For this review, take the finished solid that the model builds, in its own axes (mm). Face numbers are marked on the shaded views. A direction names the side the tool comes from. Round coordinates to 2 decimals unless told otherwise and drop trailing zeros. Loops run counter-clockwise (first coordinate to the right, second up) from the corner with the lowest first, then second, coordinate; pieces in that order, holes last.
1) Take a section at A-A (x = 77). State the section outline as (y, z) points (3 decimals).
2) Wall thickness on L1, parallel to X at y = 203, z = 24.5; L2, parallel to Z at x = 143, y = 218.5; L3, parallel to Y at x = 37, z = 125.5: over which ranges is each line inside the solid? List them lowest first.
3) Insertion check: pin 1 (2 mm diameter, centred on x = 94.5, z = 6.5, fed in from -Y); pin 2 (12 mm diameter, centred on x = 132, y = 16.5, fed in from -Z); pin 3 (4 mm diameter, centred on x = 144, y = 40.5, fed in from -Z). Each pin has a flat end and moves straight along its axis. Give the tip position at first contact, or say it passes through.
4) Mouldability with a two-part tool opening along X and no side actions: class the marked faces 1, 2 and 3 as pulls with the +X half, pulls with the -X half, needs draft (parallel to the pull), parting line crosses it, or undercut.
5) Take a section at C-C (z = 112.5). State the section outline as (x, y) points, then the cut area to 3 significant figures.
6) Take a section at B-B (z = 40). State the section outline as (x, y) points.
7) Take a section at D-D (y = 0). State the section outline as (x, z) points.
8) Tool access review of the marked faces 4, 5 and 6: name each direction out of +Z, -Z, +X, -X, +Y, -Y from which nothing blocks a thin tool from reaching the whole face with its end or side.
```python
from build123d import *

# Parameters (mm, degrees)
F0_R      = 9.5
F1_DEPTH  = 291
F3_DEPTH  = 60
F4_DEPTH  = 20
F7_DEPTH  = 20
F8_DEPTH  = 20
F10_DEPTH = 105
F11_W     = 120
F11_H     = 70
F12_DEPTH = 149.5


with BuildPart() as f1:
    # F0 (on Right) → F1 (new body)
    with BuildSketch(Plane.YZ):
        Circle(F0_R)
    extrude(amount=F1_DEPTH)

    # F2 (on Front) → F3 (join)
    with BuildSketch(Plane.XZ):
        Polygon((125, -2.5), (145, -2.5), (145, 2.5), (125, 2.5), (125, 0), align=None)
    extrude(amount=F3_DEPTH)

    # F2 (on Front) → F4 (join)
    with BuildSketch(Plane.XZ):
        Polygon((125, -2.5), (145, -2.5), (145, 2.5), (125, 2.5), (125, 0), align=None)
    extrude(amount=-F4_DEPTH)

    # F6 (on offset) → F7 (join)
    with BuildSketch(Plane.YZ.offset(125)):
        Polygon((20, 2.5), (20, 0), (20, -2.5), (82.621394, 128.280584), (82.341, 132.695), align=None)
    extrude(amount=F7_DEPTH)

    # F6 (on offset) → F8 (join)
    with BuildSketch(Plane.YZ.offset(125)):
        Polygon((20, 2.5), (20, 0), (20, -2.5), (82.621394, 128.280584), (82.341, 132.695), align=None)
        Polygon((181.532421, 54.58217), (82.341, 132.695), (82.621394, 128.280584), (181.532421, 50.388562), align=None)
        Polygon((256.532421, 54.58217), (181.532421, 54.58217), (181.532421, 50.388562), (181.532421, -0.41783), (256.532421, -0.41783), align=None)
    extrude(amount=F8_DEPTH)

    # F9 (on face) → F10 (join)
    with BuildSketch(Plane(origin=(125, 0, 0), x_dir=(0, -1, 0), z_dir=(-1, 0, 0))):
        Polygon((-181.532421, 54.58217), (-256.532421, 54.58217), (-256.532421, -0.41783), (-181.532421, -0.41783), (-181.532421, 50.388562), align=None)
        Polygon((-82.341, 132.695), (-181.532421, 54.58217), (-181.532421, 50.388562), (-82.621394, 128.280584), align=None)
    extrude(amount=F10_DEPTH)

    # F11 (on face) → F12 (cut)
    with BuildSketch(Plane.XY.offset(54.58217)):
        with Locations((82.5, 219.032421)):
            Rectangle(F11_W, F11_H)
    extrude(amount=-F12_DEPTH, mode=Mode.SUBTRACT)


solid = f1.part
```
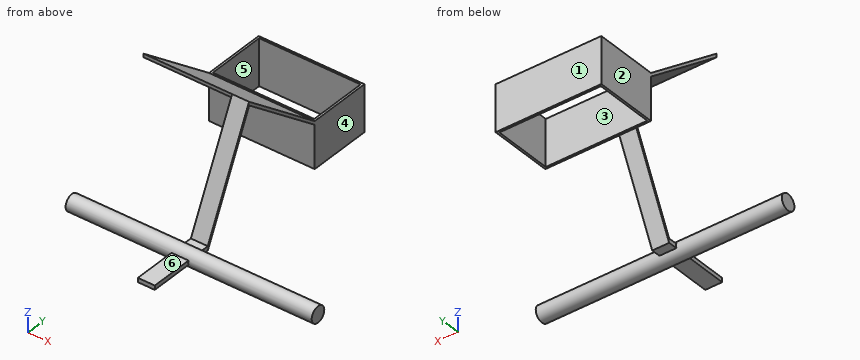
Response:
1. outline: circle Ø19 at (0, 0); (82.341, 132.695) - (82.621, 128.281) - (181.532, 50.389) - (181.532, -0.418) - (184.032, -0.418) - (184.032, 54.582) - (181.532, 54.582) - close; (254.032, -0.418) - (256.532, -0.418) - (256.532, 54.582) - (254.032, 54.582) - close
2. L1: x = 20 to 22.5, 142.5 to 145
2. L2: z = -0.42 to 54.58
2. L3: y = 86.15 to 91.48
3. pin 1: stops at y = -7.75
3. pin 2: stops at z = -2.5
3. pin 3: stops at z = 36.14
4. face 1: needs draft
4. face 2: pulls with the -X half
4. face 3: undercut
5. outline: (20, 102.66) - (145, 102.66) - (145, 107.99) - (20, 107.99) - close; (125, 72.67) - (145, 72.67) - (145, 75.07) - (125, 75.07) - close
5. area: 714 mm2
6. outline: (20, 181.53) - (145, 181.53) - (145, 256.53) - (20, 256.53) - close; (125, 37.96) - (145, 37.96) - (145, 40.35) - (125, 40.35) - close; hole (22.5, 184.03) - (142.5, 184.03) - (142.5, 254.03) - (22.5, 254.03) - close
7. outline: (0, -9.5) - (291, -9.5) - (291, 9.5) - (0, 9.5) - close
8. face 4: +Z, -Z, +X, +Y
8. face 5: +Z, -Z
8. face 6: +Z, +X, -X, -Y
